Work out the finished part from the listing and answer in its coordinate system (mm). A direction names the side the tool comes from. Round coordinates to 2 decimals unless told otherwise and drop trailing zeros. Write each loop counter-clockwise with the first axis right and the second up, starting at its lowest first coordinate (ties: lowest second). Pieces come first, ordered by that corner, then holes.
1. Straight lines are drawn through the part: probe 1 along Z at (x, y) = (0, 37.75); probe 2 along Z at (x, y) = (0, 6.5); probe 3 along X at (y, z) = (39.25, 0). For each, find the intervals that lie inside material, in ascending order.
2. Find section A-A (z = 0). Write down the section's boundary in (x, y).
3. Find section B-B (y = 10). Write down the section's boundary in (x, z), and give its area (3 significant figures).
4. Find section D-D (y = 35.5). Write down the section's boundary in (x, z).
5. Find section C-C (x = -1). Write down the section's boundary in (y, z).
6. Flat-ended cylindrical pins translate along their axes: pin 1 Ø3 at (x, z) = (-2, 1) entering from +Y; pin 2 Ø1 at (x, y) = (-2, 14) entering from -Z; pin 3 Ø3 at (x, z) = (0, 0) entering from +Y; pin 4 Ø2 at (y, z) = (31.5, -6) entering from -X. Find the tip coordinate at first contact, or state that the pin passes through.
7. A tool of negligible diameter and unlimited length cuts with its end or side. For faces 1 (the face through (2, 0, -2)), 2 (the face through (2, 27.7, -1)), from which of +Z, -Z, +X, -X, +Y, -Y can it reach the whole face along a straight path? Write none if from no direction.
8. Determine the mould class of faces 3 (the face through (3.219, 23.048, 5.474)), 4 (the face through (-6.35, 23, 0)), 5 (the face through (2.435, 37.358, -0.767)) for opening direction Z: pulls with the +Z half, pulls with the -Z half, needs draft (parallel to the pull), parting line crosses it, or undercut.
Autodesk Inventor part; units mm, degrees
ref_plane "YZ Plane" through (0, 0, 0) normal (1, 0, 0) x (0, 1, 0)
ref_plane "XZ Plane" through (0, 0, 0) normal (0, 1, 0) x (-1, 0, 0)
ref_plane "XY Plane" through (0, 0, 0) normal (0, 0, 1) x (1, 0, 0)
sketch "Sketch1" plane through (0, 0, 0) normal (0, 1, 0) x (-1, 0, 0)
  line L0 (6.35, 3.6662) -> (6.35, -3.6662)
  line L1 (6.35, -3.6662) -> (0, -7.3323)
  line L2 (0, -7.3323) -> (-6.35, -3.6662)
  line L3 (-6.35, -3.6662) -> (-6.35, 3.6662)
  line L4 (-6.35, 3.6662) -> (0, 7.3323)
  line L5 (0, 7.3323) -> (6.35, 3.6662)
  point P0 (0, 0)
  point P1 (0, 0)
  dimension "d0" = 12.7
extrude "Extrusion1" add sketch "Sketch1" along normal blind 46.75
sketch "Sketch2" plane through (0, 46.75, 0) normal (0, 1, 0) x (1, 0, 0)
  circle A0 centre (0, 0) radius 2.5527
  dimension "d3" = 5.1054
extrude "Extrusion2" cut sketch "Sketch2" against normal blind 19.05
sketch "Sketch3" plane through (0, 0, 0) normal (0, -1, 0) x (1, 0, 0)
  circle A0 centre (0, 0) radius 2.0193
  dimension "d6" = 4.0386
extrude "Extrusion3" cut sketch "Sketch3" against normal through all
thread "Thread1"
thread "Thread2"
properties part number "CORL_013_SmallShaft" material "Aluminum 6061"
Worked answers:
1. probe 1: z = -7.33 to -2.55, 2.55 to 7.33
1. probe 2: z = -7.33 to -2.02, 2.02 to 7.33
1. probe 3: x = -6.35 to -2.55, 2.55 to 6.35
2. outline: (-6.35, 0) - (-2.02, 0) - (-2.02, 27.7) - (-2.55, 27.7) - (-2.55, 46.75) - (-6.35, 46.75) - close; (2.02, 0) - (6.35, 0) - (6.35, 46.75) - (2.55, 46.75) - (2.55, 27.7) - (2.02, 27.7) - close
3. outline: (-6.35, -3.67) - (0, -7.33) - (6.35, -3.67) - (6.35, 3.67) - (0, 7.33) - (-6.35, 3.67) - close; hole circle Ø4.04 at (0, 0)
3. area: 127 mm2
4. outline: (-6.35, -3.67) - (0, -7.33) - (6.35, -3.67) - (6.35, 3.67) - (0, 7.33) - (-6.35, 3.67) - close; hole circle Ø5.11 at (0, 0)
5. outline: (0, -6.75) - (46.75, -6.75) - (46.75, -2.35) - (27.7, -2.35) - (27.7, -1.75) - (0, -1.75) - close; (0, 1.75) - (27.7, 1.75) - (27.7, 2.35) - (46.75, 2.35) - (46.75, 6.75) - (0, 6.75) - close
6. pin 1: stops at y = 46.75
6. pin 2: stops at z = -6.47
6. pin 3: passes through
6. pin 4: stops at x = -4.04
7. face 1: +Z, -Z, +X, -X, -Y
7. face 2: +Y
8. face 3: pulls with the +Z half
8. face 4: needs draft
8. face 5: undercut
